Geometry check sheet. Reference: the model listing, model coordinates, mm. A direction names the side the tool comes from. Coordinates: 2 decimals unless noted, no trailing zeros. Loops run counter-clockwise (first coordinate to the right, second up) from the corner with the lowest first, then second, coordinate; pieces in that order, holes last. Notation, with made-up numbers: (30, 30) - (81, 30) arc R25 cw to (81, 56) - close; hole circle Ø1 at (22.25, -21). An arc over 180 degrees is marked (long way). Write each question's results on one line, items separated by ' | '. Start each with the question number.
(1) Sectioned sample at D-D (x = -5.25). Enter the section's corners in (y, z).
(2) Access from +Z, -Z, +X, -X, +Y, -Y to the whole of each face (thin tool, end or side, straight path). Record for faces 1 (the face through (3, 22, -12)), 2 (the face through (-1.97, 50.11, -16.52)), 3 (the face through (-8, 54, -12)).
(3) Sectioned sample at B-B (x = 4). Enter the section's corners in (y, z), plus the area to 3 significant figures.
(4) Material ranges on probe 1 along Y at (x, z) = (-6.4, -17.5); probe 2 along Y at (x, z) = (-1.65, -17.5); probe 3 along X at (y, z) = (29, -19.5), recorded low to high.
(5) Mould release check, pull along Y, two halves, no side actions. Record for faces 4 (the face through (6, 9, -12)), 5 (the face through (-4, 52.6, -9.4)), 6 (the face through (-4, 52.6, -19.4)), 7 (the face through (-1, 109, -12)): pulls with the +Y half, pulls with the -Y half, needs draft (parallel to the pull), parting line crosses it, or undercut.
(6) Go/stop test with flat-tipped pins: pin 1 Ø6 at (y, z) = (59.5, -3.5) entering from +X; pin 2 Ø4.5 at (y, z) = (54.5, -18) entering from +X. Record where each tip stops, or that it passes through.
(7) Sectioned sample at C-C (y = 54.5). Enter the section's corners in (x, z), plus the area to 3 significant figures.
(8) Sectioned sample at A-A (y = 13.5). Enter the section's corners in (x, z).
Autodesk Inventor part; units mm, degrees
ref_plane "YZ Plane" through (0, 0, 0) normal (1, 0, 0) x (0, 1, 0)
ref_plane "XZ Plane" through (0, 0, 0) normal (0, 1, 0) x (-1, 0, 0)
ref_plane "XY Plane" through (0, 0, 0) normal (0, 0, 1) x (1, 0, 0)
sketch "Sketch1" plane through (0, 0, 0) normal (0, 1, 0) x (-1, 0, 0)
  line L0 (0, 0) -> (8, 0)
  line L1 (8, 0) -> (8, -25)
  line L2 (8, -25) -> (0, -25)
  line L3 (0, -25) -> (0, 0)
  dimension "d0" = 8
  dimension "d1" = 25
extrude "Extrusion1" add sketch "Sketch1" along normal blind 109
sketch "Sketch2" plane through (0, 0, 0) normal (1, 0, 0) x (0, 0, -1)
  line L0 (0, 109) -> (25, 109)
  line L1 (0, 109) -> (25, 109)
  line L2 (25, 109) -> (25, 87)
  line L3 (25, 87) -> (0, 87)
  line L4 (0, 87) -> (0, 109)
  line L5 (25, 0) -> (25, 109)
  line L6 (25, 0) -> (0, 0)
  line L7 (0, 0) -> (0, 22)
  line L8 (0, 22) -> (25, 22)
  line L9 (25, 22) -> (25, 0)
  dimension "d4" = 25
  dimension "d5" = 22
  dimension "d6" = 25
  dimension "d7" = 22
extrude "Extrusion2" add sketch "Sketch2" along normal blind 6
sketch "Sketch3" plane through (6, 0, 0) normal (1, 0, 0) x (0, 0, -1)
  line L0 (0, 0) -> (25, 0)
  line L1 (0, 0) -> (12.5, 0)
  line L2 (12.5, 0) -> (12.5, 13.5)
  circle A0 centre (12.5, 13.5) radius 3.5
  circle A1 centre (12.5, 95.5) radius 3.5
  line L3 (25, 109) -> (0, 109)
  line L4 (0, 109) -> (0, 87)
  dimension "d10" = 13.5
  dimension "d11" = 7
  dimension "d12" = 7
  dimension "d13" = 13.5
  dimension "d14" = 12.5
sketch "Sketch4" plane through (0, 22, -25) normal (1, 0, 0) x (0, 0, -1)
  circle A0 centre (-17.5, 32.5) radius 2.5
  line L0 (-25, -22) -> (0, -22)
  line L1 (-25, 0) -> (-25, 65)
  circle A1 centre (-7.5, 32.5) radius 2.5
  line L2 (0, 0) -> (0, 65)
  circle A2 centre (-12.5, 22.5) radius 2.5
  circle A3 centre (-12.5, 42.5) radius 2.5
  dimension "d15" = 5
  dimension "d16" = 54.5
  dimension "d17" = 7.5
  dimension "d18" = 5
  dimension "d19" = 7.5
  dimension "d20" = 54.5
  dimension "d21" = 5
  dimension "d22" = 5
  dimension "d23" = 10
  dimension "d24" = 5
  dimension "d25" = 10
  dimension "d26" = 5
extrude "Extrusion3" cut sketch "Sketch3" against normal up to next
extrude "Extrusion4" cut sketch "Sketch4" against normal up to next
sketch "Sketch5" plane through (0, 22, -25) normal (1, 0, 0) x (0, 0, -1)
  circle A0 centre (-12.5, 42.5) radius 2.5
  circle A1 centre (-12.5, 42.5) radius 4.5
  circle A2 centre (-17.5, 32.5) radius 2.5
  circle A3 centre (-17.5, 32.5) radius 4.5
  circle A4 centre (-7.5, 32.5) radius 2.5
  circle A5 centre (-7.5, 32.5) radius 4.5
  circle A6 centre (-12.5, 22.5) radius 2.5
  circle A7 centre (-12.5, 22.5) radius 4.5
  point P0 (-25, -22)
  dimension "d31" = 9
  dimension "d32" = 9
  dimension "d33" = 9
  dimension "d34" = 9
extrude "Extrusion5" cut sketch "Sketch5" against normal blind 4
properties part number "Back_Bracket" material "ABS Plastic"
Outcome:
1) outline: (0, -25) - (109, -25) - (109, 0) - (0, 0) - close; hole circle Ø7 at (13.5, -12.5); hole circle Ø5 at (44.5, -12.5); hole circle Ø5 at (54.5, -17.5); hole circle Ø5 at (54.5, -7.5); hole circle Ø5 at (64.5, -12.5); hole circle Ø7 at (95.5, -12.5)
2) face 1: +Z, -Z, +X | face 2: +X | face 3: +Z, -Z, -X, +Y, -Y
3) outline: (0, -25) - (22, -25) - (22, 0) - (0, 0) - close; (87, -25) - (109, -25) - (109, 0) - (87, 0) - close; hole circle Ø7 at (13.5, -12.5); hole circle Ø7 at (95.5, -12.5) | area: 1,020 mm2
4) probe 1: y = 0 to 52, 57 to 109 | probe 2: y = 0 to 50, 59 to 109 | probe 3: x = -8 to 0
5) face 4: needs draft | face 5: undercut | face 6: undercut | face 7: pulls with the +Y half
6) pin 1: stops at x = 0 | pin 2: stops at x = -4
7) outline: (-8, -25) - (0, -25) - (0, -22) - (-4, -22) - (-4, -20) - (-8, -20) - close; (-8, -15) - (-4, -15) - (-4, -13) - (0, -13) - (0, -12) - (-4, -12) - (-4, -10) - (-8, -10) - close; (-8, -5) - (-4, -5) - (-4, -3) - (0, -3) - (0, 0) - (-8, 0) - close | area: 88.0 mm2
8) outline: (-8, -25) - (6, -25) - (6, -16) - (-8, -16) - close; (-8, -9) - (6, -9) - (6, 0) - (-8, 0) - close
